CAD build for the part. Positions are in the model's coordinates, mm. A direction names the side the tool comes from. Round coordinates to 2 decimals unless told otherwise and drop trailing zeros. Write each loop counter-clockwise with the first axis right and the second up, starting at its lowest first coordinate (ties: lowest second). Pieces come first, ordered by that corner, then holes. Notation, with made-up numbers: (46.25, 2) - (60.25, 2) arc R19 cw to (60.25, 35) - close; hole circle Ø6 at (-27, 66). An arc over 180 degrees is marked (long way). Put each result on its own line as item: value. Start each with the question number.
Item 1: Cut at A-A (z = -14). Give the cut face in (x, y), and give its area (3 significant figures).
Item 2: Drill centre lines: line 1 (X direction, y = 0.7, z = 2); line 2 (Z direction, x = 14, y = 0.55); line 3 (X direction, y = 4.5, z = -28.5). Where is each one in solid material? Low to high. Write a range as from..to.
Item 3: Cut at D-D (y = 4.9). Count the separate pieces of the cut face and the enclosed holes in it, and give its area (3 significant figures).
Item 4: 3-axis set-ups, long thin cutter, end or side, ignore diameter. For faces 1 (the flat face through (-23, 3, -25.285)), 2 (the flat face through (-12.924, 3, -17)), 3 (the flat face through (22.076, 3, -28)): which of +Z, -Z, +X, -X, +Y, -Y reach the whole face in a straight line?
Item 5: Cut at C-C (x = 23.5). Give the cut face in (y, z).
Item 6: Mould opens along X. For faces 4 (the cylindrical face through (2.83, 2.96, 7.1)), 5 (the flat face through (-17.924, 3, -28)), 6 (the flat face through (2, 6, -7)) say: released by +X, released by -X, zero draft, split by the parting line, or undercut.
Item 7: Cut at B-B (z = 3). Give the cut face in (x, y).
Item 8: Pin check, flat tips, straight feed: pin 1 Ø12 at (x, z) = (-11.5, 10) entering from -Y; pin 2 Ø4 at (x, z) = (2.08, 4.72) entering from +Y. Stop position of each tip, or through.
```python
from build123d import *

# Parameters (mm, degrees)
SKETCH2_R           = 2.5
SKETCH2_W           = 5
SKETCH2_H           = 10
BOSS_EXTRUDE1_DEPTH = 6


with BuildPart() as part:
    # Sketch2 → Boss-Extrude1 (new body)
    with BuildSketch(Plane(origin=(0, 0, 0), x_dir=(1, 0, 0), z_dir=(0, 1, 0))):
        Polygon((-27.923792882, 25.284964835), (-17.923792882, 25.284964835), (-17.923792882, 31.284964835), (-7.923792882, 31.284964835), (-7.923792882, 25.284964835), (12.076207118, 25.284964835), (12.076207118, 31.284964835), (22.076207118, 31.284964835), (22.076207118, 25.284964835), (32.076207118, 25.284964835), (32.076207118, -18.715035165), (-27.923792882, -18.715035165), align=None)
        with Locations(Location((2.076207118, 17.284964835, 0), (0, 0, 270))):
            Circle(SKETCH2_R, mode=Mode.SUBTRACT)
        with Locations(Location((2.076207118, -4.715035165, 0), (0, 0, 270))):
            Circle(SKETCH2_R, mode=Mode.SUBTRACT)
        with Locations((-10.423792882, -4.715035165)):
            Rectangle(SKETCH2_W, SKETCH2_H, mode=Mode.SUBTRACT)
        with Locations((-10.423792882, 17.284964835)):
            Rectangle(SKETCH2_W, SKETCH2_H, mode=Mode.SUBTRACT)
        with Locations((14.576207118, 17.284964835)):
            Rectangle(SKETCH2_W, SKETCH2_H, mode=Mode.SUBTRACT)
        with Locations((14.576207118, -4.715035165)):
            Rectangle(SKETCH2_W, SKETCH2_H, mode=Mode.SUBTRACT)
    extrude(amount=BOSS_EXTRUDE1_DEPTH)


solid = part.part
```
Output values:
1. outline: (-27.92, 0) - (-12.92, 0) - (-12.92, 6) - (-27.92, 6) - close; (-7.92, 0) - (12.08, 0) - (12.08, 6) - (-7.92, 6) - close; (17.08, 0) - (32.08, 0) - (32.08, 6) - (17.08, 6) - close
1. area: 300 mm2
2. line 1: -27.92..-12.92, -7.92..12.08, 17.08..32.08
2. line 2: -31.28..-22.28, -12.28..-0.28, 9.72..18.72
2. line 3: -17.92..-7.92, 12.08..22.08
3. separate pieces: 1
3. enclosed holes: 6
3. area: 2,520 mm2
4. face 1: -Z, -X, +Y, -Y
4. face 2: +Y, -Y
4. face 3: -Z, +X, +Y, -Y
5. outline: (0, -25.28) - (6, -25.28) - (6, 18.72) - (0, 18.72) - close
6. face 4: undercut
6. face 5: released by -X
6. face 6: zero draft
7. outline: (-27.92, 0) - (-12.92, 0) - (-12.92, 6) - (-27.92, 6) - close; (-7.92, 0) - (0.26, 0) - (0.26, 6) - (-7.92, 6) - close; (3.9, 0) - (12.08, 0) - (12.08, 6) - (3.9, 6) - close; (17.08, 0) - (32.08, 0) - (32.08, 6) - (17.08, 6) - close
8. pin 1: y = 0
8. pin 2: through
